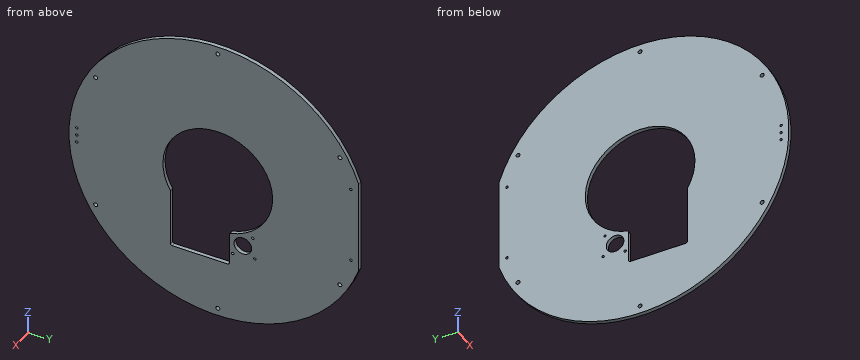
```python
from build123d import *

# Parameters (mm, degrees)
SKETCH1_R           = 3.2639
SKETCH1_R_2         = 2.0193
SKETCH1_R_3         = 14.2875
BOSS_EXTRUDE1_DEPTH = 6.35
FILLET1_R           = 2.54


with BuildPart() as part:
    # Sketch1 → Boss-Extrude1 (new body)
    with BuildSketch(Plane(origin=(0, 0, 0), x_dir=(0, 0, -1), z_dir=(1, 0, 0))):
        with BuildLine():
            Line((77.251084135, 228.6), (-77.251084135, 228.6))
            ThreePointArc((-77.251084135, 228.6), (0, -241.3), (77.251084135, 228.6))
        make_face()
        with Locations((-114.3, -197.973407305)):
            Circle(SKETCH1_R, mode=Mode.SUBTRACT)
        with Locations((-12.7, -228.6)):
            Circle(SKETCH1_R_2, mode=Mode.SUBTRACT)
        with Locations((0, -228.6)):
            Circle(SKETCH1_R_2, mode=Mode.SUBTRACT)
        with Locations((12.7, -228.6)):
            Circle(SKETCH1_R_2, mode=Mode.SUBTRACT)
        with Locations((114.3, -197.973407305)):
            Circle(SKETCH1_R, mode=Mode.SUBTRACT)
        with Locations((228.6, 0)):
            Circle(SKETCH1_R, mode=Mode.SUBTRACT)
        with Locations((-228.6, 0)):
            Circle(SKETCH1_R, mode=Mode.SUBTRACT)
        with Locations((-114.3, 197.973407305)):
            Circle(SKETCH1_R, mode=Mode.SUBTRACT)
        with Locations((-63.5, 215.9)):
            Circle(SKETCH1_R_2, mode=Mode.SUBTRACT)
        with BuildLine():
            Line((142.875, -76.522457682), (45.249568731, -76.522457682))
            ThreePointArc((45.249568731, -76.522457682), (-81.451531518, 35.6210333), (86.905058303, 18.727542318))
            Line((86.905058303, 18.727542318), (142.875, 18.727542318))
            Line((142.875, 18.727542318), (142.875, -76.522457682))
        make_face(mode=Mode.SUBTRACT)
        with Locations((82.142471145, 56.966805286)):
            Circle(SKETCH1_R_2, mode=Mode.SUBTRACT)
        with Locations((101.6, 40.64)):
            Circle(SKETCH1_R_3, mode=Mode.SUBTRACT)
        with Locations((117.926805286, 60.097528855)):
            Circle(SKETCH1_R_2, mode=Mode.SUBTRACT)
        with Locations((121.057528855, 24.313194714)):
            Circle(SKETCH1_R_2, mode=Mode.SUBTRACT)
        with Locations((114.3, 197.973407305)):
            Circle(SKETCH1_R, mode=Mode.SUBTRACT)
        with Locations((63.5, 215.9)):
            Circle(SKETCH1_R_2, mode=Mode.SUBTRACT)
    extrude(amount=BOSS_EXTRUDE1_DEPTH)

    # Fillet1
    fillet1_edges = [part.edges().sort_by_distance(p)[0] for p in [
        (3.175, -76.522457682, -45.249568731),
        (3.175, -76.522457682, -142.875),
        (3.175, 18.727542318, -142.875),
        (3.175, 18.727542318, -86.905058303),
    ]]
    fillet(fillet1_edges, radius=FILLET1_R)


solid = part.part
```
Check sheet for the modelled part. Datum: model origin and axes. Units: mm. Coordinates: 2 decimals unless noted, no trailing zeros. Loops run counter-clockwise (first coordinate to the right, second up) from the corner with the lowest first, then second, coordinate; pieces in that order, holes last.
1) Sectioned sample at C-C (z = -101.6). Record the boundary of the cut face in (x, y), and give its area (3 significant figures).
2) Material ranges on probe 1 along Y at (x, z) = (3.5, 114.3); probe 2 along Y at (x, z) = (2.5, -114.3); probe 3 along Y at (x, z) = (4.5, 12.7), recorded low to high.
3) Sectioned sample at D-D (y = 158). Record the boundary of the cut face in (x, z).
4) Sectioned sample at A-A (z = 50). Record the boundary of the cut face in (x, y), and give its area (3 significant figures).
5) Gauge pin test, flat ends, axial feed: pin 1 (7.5 mm diameter, centred on y = -197.97, z = 114.3, fed in from +X); pin 2 (1.9 mm diameter, centred on x = 4.5, z = -82.5, fed in from +Y); pin 3 (5 mm diameter, centred on y = 0, z = -228.6, fed in from -X); pin 4 (1.9 mm diameter, centred on x = 3, z = -116, fed in from -Y). Record the tip position at first contact, or that the pin passes through.
6) Sectioned sample at B-B (x = 2.25). Count the separate pieces of the cut face and the enclosed holes in it, and give its area (3 significant figures).
Check sheet entries:
1. outline: (0, -218.87) - (6.35, -218.87) - (6.35, -76.52) - (0, -76.52) - close; (0, 18.73) - (6.35, 18.73) - (6.35, 26.35) - (0, 26.35) - close; (0, 54.93) - (6.35, 54.93) - (6.35, 218.87) - (0, 218.87) - close
1. area: 1,990 mm2
2. probe 1: y = -212.51 to -201.24, -194.71 to 194.71, 201.24 to 212.51
2. probe 2: y = -212.51 to -201.24, -194.71 to -76.52, 18.73 to 34.09, 47.19 to 194.71, 201.24 to 212.51
2. probe 3: y = -240.97 to -230.62, -226.58 to -87.99, 87.99 to 228.6
3. outline: (0, -182.38) - (6.35, -182.38) - (6.35, 182.38) - (0, 182.38) - close
4. outline: (0, -236.06) - (6.35, -236.06) - (6.35, -73.51) - (0, -73.51) - close; (0, 73.51) - (6.35, 73.51) - (6.35, 228.6) - (0, 228.6) - close
4. area: 2,020 mm2
5. pin 1: stops at x = 6.35
5. pin 2: stops at y = 227.1
5. pin 3: passes through
5. pin 4: stops at y = -212.11
6. separate pieces: 1
6. enclosed holes: 16
6. area: 150,000 mm2
